```python
from build123d import *

# Parameters (mm, degrees)
SKETCH1_R           = 1.5
BOSS_EXTRUDE1_DEPTH = 2
SKETCH4_W           = 25
SKETCH4_H           = 35
SKETCH4_W_2         = 35
BOSS_EXTRUDE4_DEPTH = 2
BOSS_EXTRUDE5_START = -2
BOSS_EXTRUDE5_DEPTH = 2


with BuildPart() as part:
    # Sketch1 → Boss-Extrude1 (new body)
    with BuildSketch(Plane.XY):
        Polygon((-480, 80), (-455, 80), (-455, -80), (-443, -80), (-443, 80), (-418, 80), (-418, -80), (-406, -80), (-406, 80), (-381, 80), (-381, -80), (-369, -80), (-369, 80), (-344, 80), (-344, -80), (-332, -80), (-332, 80), (-307, 80), (-307, -80), (-295, -80), (-295, 80), (-270, 80), (-270, -80), (-258, -80), (-258, 80), (-233, 80), (-233, -80), (-221, -80), (-221, 80), (-196, 80), (-196, -80), (-184, -80), (-184, 80), (-159, 80), (-159, -80), (-147, -80), (-147, 80), (-122, 80), (-122, -80), (-110, -80), (-110, 80), (-85, 80), (-85, -80), (-73, -80), (-73, 80), (-48, 80), (-48, -80), (-36, -80), (-36, 80), (-11, 80), (-11, -80), (1, -80), (1, 80), (26, 80), (26, -80), (38, -80), (38, 80), (63, 80), (63, -80), (75, -80), (75, 80), (100, 80), (100, -80), (112, -80), (112, 80), (137, 80), (137, -80), (149, -80), (149, 80), (174, 80), (174, -80), (186, -80), (186, 80), (211, 80), (211, -80), (223, -80), (223, 80), (248, 80), (248, -80), (260, -80), (260, 80), (285, 80), (285, -80), (297, -80), (297, 80), (322, 80), (322, -80), (334, -80), (334, 80), (359, 80), (359, -80), (371, -80), (371, 80), (396, 80), (396, -80), (408, -80), (408, 80), (433, 80), (433, -80), (445, -80), (445, 80), (480, 80), (480, -100), (-480, -100), align=None)
        with Locations((0, -95)):
            Circle(SKETCH1_R, mode=Mode.SUBTRACT)
    extrude(amount=BOSS_EXTRUDE1_DEPTH)

    # Sketch4 → Boss-Extrude4 (add)
    with BuildSketch(Plane(origin=(0, 80, 0), x_dir=(1, 0, 0), z_dir=(0, 1, 0))):
        with Locations((-430.5, 17.5)):
            Rectangle(SKETCH4_W, SKETCH4_H)
        with Locations((-467.5, 17.5)):
            Rectangle(SKETCH4_W, SKETCH4_H)
        with Locations((-393.5, 17.5)):
            Rectangle(SKETCH4_W, SKETCH4_H)
        with Locations((-356.5, 17.5)):
            Rectangle(SKETCH4_W, SKETCH4_H)
        with Locations((-319.5, 17.5)):
            Rectangle(SKETCH4_W, SKETCH4_H)
        with Locations((-282.5, 17.5)):
            Rectangle(SKETCH4_W, SKETCH4_H)
        with Locations((-245.5, 17.5)):
            Rectangle(SKETCH4_W, SKETCH4_H)
        with Locations((-208.5, 17.5)):
            Rectangle(SKETCH4_W, SKETCH4_H)
        with Locations((-171.5, 17.5)):
            Rectangle(SKETCH4_W, SKETCH4_H)
        with Locations((-134.5, 17.5)):
            Rectangle(SKETCH4_W, SKETCH4_H)
        with Locations((-97.5, 17.5)):
            Rectangle(SKETCH4_W, SKETCH4_H)
        with Locations((-60.5, 17.5)):
            Rectangle(SKETCH4_W, SKETCH4_H)
        with Locations((-23.5, 17.5)):
            Rectangle(SKETCH4_W, SKETCH4_H)
        with Locations((13.5, 17.5)):
            Rectangle(SKETCH4_W, SKETCH4_H)
        with Locations((50.5, 17.5)):
            Rectangle(SKETCH4_W, SKETCH4_H)
        with Locations((87.5, 17.5)):
            Rectangle(SKETCH4_W, SKETCH4_H)
        with Locations((124.5, 17.5)):
            Rectangle(SKETCH4_W, SKETCH4_H)
        with Locations((161.5, 17.5)):
            Rectangle(SKETCH4_W, SKETCH4_H)
        with Locations((198.5, 17.5)):
            Rectangle(SKETCH4_W, SKETCH4_H)
        with Locations((235.5, 17.5)):
            Rectangle(SKETCH4_W, SKETCH4_H)
        with Locations((272.5, 17.5)):
            Rectangle(SKETCH4_W, SKETCH4_H)
        with Locations((309.5, 17.5)):
            Rectangle(SKETCH4_W, SKETCH4_H)
        with Locations((346.5, 17.5)):
            Rectangle(SKETCH4_W, SKETCH4_H)
        with Locations((383.5, 17.5)):
            Rectangle(SKETCH4_W, SKETCH4_H)
        with Locations((420.5, 17.5)):
            Rectangle(SKETCH4_W, SKETCH4_H)
        with Locations((462.5, 17.5)):
            Rectangle(SKETCH4_W_2, SKETCH4_H)
    extrude(amount=-BOSS_EXTRUDE4_DEPTH)

    # Sketch5 → Boss-Extrude5 (add)
    with BuildSketch(Plane.XY.offset(2).offset(BOSS_EXTRUDE5_START)):
        with BuildLine():
            Line((0, -95), (0.513030215, -93.590461069))
            ThreePointArc((0.513030215, -93.590461069), (0, -93.5), (-0.513030215, -93.590461069))
            Line((-0.513030215, -93.590461069), (0, -95))
        make_face()
    extrude(amount=BOSS_EXTRUDE5_DEPTH)


solid = part.part
```
The listing builds one solid part. Answer for the finished solid, in the listing's coordinates (mm). A direction names the side the tool comes from. Coordinates: 2 decimals unless noted, no trailing zeros. Write each loop counter-clockwise with the first axis right and the second up, starting at its lowest first coordinate (ties: lowest second). Pieces come first, ordered by that corner, then holes. Notation, with made-up numbers: (69, 58.5) -> (112, 58.5) arc R18 cw to (112, 90.5) -> close; hole circle Ø3 at (43.5, 80). An arc over 180 degrees is marked (long way). Write each question's results on one line, items separated by ' | '. Start each with the question number.
1) A tool of negligible diameter and unlimited length cuts with its end or side. For faces 1 (the flat face through (-320, 80, -17)), 2 (the flat face through (-381, 0, 1)), 3 (the flat face through (-209, 78, -18)), from which of +Z, -Z, +X, -X, +Y, -Y can it reach the whole face along a straight path? Write none if from no direction.
2) A cutting plane is placed at A-A (x = 201.5). Determine the outline of the cut face in (y, z), then the cut area to 3 significant figures.
3) A cutting plane is placed at B-B (z = -12). Count the separate pieces of the cut face and the enclosed holes in it, then the cut area to 3 significant figures.
4) Straight lines are drawn through the part: probe 1 along Z at (x, y) = (6, -39.5); probe 2 along Y at (x, z) = (-134, -22). For each, find the intervals that lie inside material, in ascending order.
5) Flat-ended cylindrical pins translate along their axes: pin 1 Ø1.6 at (x, z) = (-44.5, 1) entering from +Y; pin 2 Ø1 at (x, z) = (23, -17.5) entering from -Y; pin 3 Ø8 at (x, y) = (38, -27.5) entering from -Z. Find the tip coordinate at first contact, or state that the pin passes through.
6) For a pull along X with two mould halves and no side action, classify faces 4 (the flat face through (462, 78, -18)), 5 (the flat face through (26, 0, 1)), 6 (the flat face through (-369, 0, 1)) as +X half, -X half, draft (parallel to the pull), parting line (faces both ways), or undercut.
Values follow:
1) face 1: +Z, -Z, +X, -X, +Y | face 2: +Z, -Z, +Y | face 3: -Z, +X, -X, -Y
2) outline: (-100, 0) -> (78, 0) -> (78, -35) -> (80, -35) -> (80, 2) -> (-100, 2) -> close | area: 430 mm²
3) separate pieces: 26 | enclosed holes: 0 | area: 1,320 mm²
4) probe 1: 0 to 2 | probe 2: 78 to 80
5) pin 1: y = -80 | pin 2: y = 78 | pin 3: z = 0
6) face 4: draft | face 5: undercut | face 6: undercut
